Autodesk Inventor part; units mm, degrees
ref_plane "Work Plane1" through (-6, 0.6, 0.75) normal (0, 0, 1) x (1, 0, 0)
ref_plane "YZ Plane" through (0, 0, 0) normal (1, 0, 0) x (0, 1, 0)
ref_plane "XZ Plane" through (0, 0, 0) normal (0, 1, 0) x (-1, 0, 0)
sketch "Sketch1" plane through (0, 0, 0) normal (0, 1, 0) x (-1, 0, 0)
  circle A0 centre (0, 0) radius 2
  circle A1 centre (0, 0) radius 3.5
  line L0 (6, 0.75) -> (3.4187, 0.75)
  line L1 (6, 0.75) -> (6, -0.75)
  line L2 (6, -0.75) -> (3.4187, -0.75)
  line L3 (3.4187, 0.75) -> (1.854, 0.75)
  line L4 (3.2692, 1.25) -> (1.5612, 1.25)
  dimension "d0" = 4
  dimension "d1" = 1.5
  dimension "d2" = 0.75
  dimension "d3" = 0.75
  dimension "d4" = 6
  dimension "d5" = 0.5
extrude "Extrusion1" add sketch "Sketch1" along normal blind 1.5 contours A0 L3 A1 L4 | L0 L1 L2 A1 picked at (2.5643, 1.5047)
ref_plane "Work Plane1" through (-6, 0.6, 0.75) normal (0, 0, 1) x (1, 0, 0)
sketch "Sketch2" plane through (-6, 0.6, 0.75) normal (0, 0, 1) x (1, 0, 0)
  line L0 (0, 0.9) -> (0, 2.4)
  line L1 (0, 2.4) -> (1.5, 2.4)
  line L2 (1.5, 2.4) -> (1.5, 0.9)
  line L3 (0, 2.4) -> (3.875, 9.1117)
  line L4 (3.875, 9.1117) -> (5.174, 8.3617)
  line L5 (5.174, 8.3617) -> (1.5, 1.9981)
  line L6 (0, 0.9) -> (4.146, 0.9)
  point P0 (6, -0.6)
  dimension "d9" = 1.5
  dimension "d15" = 1.5
  dimension "d16" = 7
  dimension "d17" = 1.5
  dimension "d18" = 60
extrude "Extrusion2" add sketch "Sketch2" against normal blind 1.5
fillet "Fillet2" radius 0.6 16 edges at (3.4903, 1.5, -0.2609) (1.7259, 1.5, -1.0107) (1.7259, 0, -1.0107) (3.4903, 0, -0.2609) (-3.927, 0, 0.75) (-4.7093, 0, -0.75) (-3.177, 1.5, 0.75) (-6, 1.5, 0.75) (-6, 1.5, -0.75) (-4.0625, 6.3558, 0.75) (-4.0625, 6.3558, -0.75) (-4.5, 2.049, 0.75) (-4.5, 2.049, -0.75) (-2.663, 5.7799, 0.75) (-2.663, 5.7799, -0.75) (-3.9593, 1.5, -0.75)
properties part number "CUT_COPPER_Bottom_Cone_1,5mm_Connecting_Wire"
Check sheet for the modelled part. Datum: model origin and axes. Units: mm. A direction names the side the tool comes from. Coordinates: 2 decimals unless noted, no trailing zeros. Loops run counter-clockwise (first coordinate to the right, second up) from the corner with the lowest first, then second, coordinate; pieces in that order, holes last. Notation, with made-up numbers: (-20, -16.75) -> (23, -16.75) arc R12 ccw to (23, -10.75) -> close; hole circle Ø3 at (80, 78.25). An arc over 180 degrees is marked (long way). Answer in a Markdown table with one row per item.
1. Sectioned sample at A-A, the plane x = 0. Record the boundary of the cut face in (y, z), then the cut area to 3 significant figures.
Check values:
| item | result |
|---|---|
| outline | (0, -2.9) arc R0.6 ccw to (0.6, -3.5) -> (0.9, -3.5) arc R0.6 ccw to (1.5, -2.9) -> (1.5, -2.6) arc R0.6 ccw to (0.9, -2) -> (0.6, -2) arc R0.6 ccw to (0, -2.6) -> close; (0, 2.6) arc R0.6 ccw to (0.6, 2) -> (0.9, 2) arc R0.6 ccw to (1.5, 2.6) -> (1.5, 2.9) arc R0.6 ccw to (0.9, 3.5) -> (0.6, 3.5) arc R0.6 ccw to (0, 2.9) -> close |
| area | 3.88 mm2 |
2. Sectioned sample at C-C, the plane y = 2. Record the boundary of the cut face in (x, z), then the cut area to 3 significant figures.
Check values:
| item | result |
|---|---|
| outline | (-6, -0.15) arc R0.6 ccw to (-5.4, -0.75) -> (-5.1, -0.75) arc R0.6 ccw to (-4.5, -0.15) -> (-4.5, 0.15) arc R0.6 ccw to (-5.1, 0.75) -> (-5.4, 0.75) arc R0.6 ccw to (-6, 0.15) -> close |
| area | 1.94 mm2 |
3. Go/stop test with flat-tipped pins: pin 1 (2 mm diameter, centred on x = -4, y = 3, fed in from +Z); pin 2 (3 mm diameter, centred on x = -3.5, y = 2, fed in from +Z); pin 3 (1 mm diameter, centred on y = 3, z = 2, fed in from +X); pin 4 (1.7 mm diameter, centred on x = -1.5, z = 1, fed in from +Y). Record where each tip stops, or that it passes through.
Check values:
| item | result |
|---|---|
| pin 1 | stops at z = 0.75 |
| pin 2 | stops at z = 2.6 |
| pin 3 | passes through |
| pin 4 | stops at y = 9.69 |
4. Material ranges on line 1 along X through (y, z) = (0.8, 0); line 2 along Z through (x, y) = (0, 0.85); line 3 along Y through (x, z) = (-2.5, -1.25), recorded low to high. Write a range as [from, to].
Check values:
| item | result |
|---|---|
| line 1 | x = [-6, -2], [2, 3.5] |
| line 2 | z = [-3.5, -2], [2, 3.5] |
| line 3 | y = [0, 1.5] |
5. Access from +Z, -Z, +X, -X, +Y, -Y to the whole of each face (thin tool, end or side, straight path). Record for faces 1 (the face through (-2, 1, 1.25)), 2 (the face through (-2.89, 5.75, -0.58)), 3 (the face through (-2.64, 5.82, 0)), 4 (the face through (-4.09, 6.31, 0)), 5 (the face through (-2.88, 5.75, 0.57)).
Check values:
| item | result |
|---|---|
| face 1 | -X, +Y, -Y |
| face 2 | -Z, +X |
| face 3 | +Z, -Z, +X |
| face 4 | +Z, -Z, -X, +Y |
| face 5 | +Z, +X |
6. Sectioned sample at B-B, the plane z = 0. Record the boundary of the cut face in (x, y) (3 decimals).
Check values:
| item | result |
|---|---|
| outline | (-6, 0) -> (-2.6, 0) arc R0.6 ccw to (-2, 0.6) -> (-2, 0.9) arc R0.6 ccw to (-2.6, 1.5) -> (-4.5, 1.5) -> (-4.5, 2.598) -> (-0.826, 8.962) -> (-2.125, 9.712) -> (-6, 3) -> close; (2, 0.6) arc R0.6 ccw to (2.6, 0) -> (2.9, 0) arc R0.6 ccw to (3.5, 0.6) -> (3.5, 0.9) arc R0.6 ccw to (2.9, 1.5) -> (2.6, 1.5) arc R0.6 ccw to (2, 0.9) -> close |
